Model file for the job. Use its own axes, mm. A direction names the side the tool comes from. Give positions to 0.01 mm unless a question says otherwise; leave off trailing zeros. Write each loop counter-clockwise with the first axis right and the second up, starting at its lowest first coordinate (ties: lowest second). Pieces come first, ordered by that corner, then holes. Notation, with made-up numbers: (0.25, 38.5) - (30.25, 38.5) arc R14 ccw to (30.25, 42.5) - close; hole circle Ø4 at (-5.75, 84). An arc over 180 degrees is marked (long way). One line per item, written item: value. Start each with the question number.
(1) Cut at B-B, the plane x = 34. List the corners of the cut face in (y, z), and give its area (3 significant figures).
(2) 3-axis set-ups, long thin cutter, end or side, ignore diameter. For faces 1 (the face through (86, 73, 3)), 2 (the face through (46.5, -9, 3)), 3 (the face through (69, -25, 3)), 4 (the face through (76, 88, 3)): which of +Z, -Z, +X, -X, +Y, -Y reach the whole face in a straight line?
(3) Cut at C-C, the plane y = 43. List the corners of the cut face in (x, z).
(4) Probe L1, parallel to Y at x = 78, z = 5.3; L2, parallel to X at y = -9, z = 1.35; L3, parallel to X at y = 76.5, z = 3.55. List the from-to ranges inside material, lowest first.
(5) Mould opens along X. For faces 5 (the face through (36.09, 29.32, 2.96)), 6 (the face through (59, 38, 6)), 7 (the face through (81.1, 81, 3)) say: pulls with the +X half, pulls with the -X half, needs draft (parallel to the pull), parting line crosses it, or undercut.
(6) Drop flat-ended pins along their axis: P1, Ø12, axis at x = 82, y = -8.5, coming from the -Z side; P2, Ø10, axis at x = 61, y = 18.5, coming from the -Z side; P3, Ø3, axis at y = 79.5, z = 4.5, coming from the -X side; P4, Ø1.8, axis at y = -5, z = 2, coming from the -X side. Give the stop position or say it passes through.
(7) Cut at A-A, the plane z = 4.45. List the corners of the cut face in (x, y).
from build123d import *

# Parameters (mm, degrees)
BOSS_EXTRU_1_DEPTH = 6
FILLET1_R          = 5
FILLET1_2_R        = 3
FILLET1_3_R        = 1


with BuildPart() as part:
    # Esquisse1 → Boss.-Extru.1 (new body)
    with BuildSketch(Plane.XY):
        with BuildLine():
            Line((46.5, 0), (46.5, -18))
            Line((46.5, -18), (67, -25))
            Line((67, -25), (71, -25))
            Line((71, -25), (71, 88))
            Line((71, 88), (81.1, 88))
            Line((81.1, 88), (81.1, 73))
            Line((81.1, 73), (91.1, 73))
            Line((91.1, 73), (91.1, 100))
            Line((91.1, 100), (69, 100))
            Line((69, 100), (10.371982926, 45.328489608))
            ThreePointArc((10.371982926, 45.328489608), (36.363080219, 28.982346298), (46.5, 0))
        make_face()
    extrude(amount=BOSS_EXTRU_1_DEPTH)

    # Fillet1
    fillet1_edges = [part.edges().sort_by_distance(p)[0] for p in [
        (69, 100, 3),
    ]]
    fillet(fillet1_edges, radius=FILLET1_R)

    # Fillet1 2
    fillet1_2_edges = [part.edges().sort_by_distance(p)[0] for p in [
        (91.1, 100, 3),
    ]]
    fillet(fillet1_2_edges, radius=FILLET1_2_R)

    # Fillet1 3
    fillet1_3_edges = [part.edges().sort_by_distance(p)[0] for p in [
        (91.1, 73, 3),
        (81.1, 73, 3),
    ]]
    fillet(fillet1_3_edges, radius=FILLET1_3_R)


solid = part.part
Answers follow:
1. outline: (31.72, 0) - (67.36, 0) - (67.36, 6) - (31.72, 6) - close
1. area: 214 mm²
2. face 1: +Z, -Z, +X, -Y
2. face 2: +Z, -Z, -X, -Y
2. face 3: +Z, -Z, +X, -X, -Y
2. face 4: +Z, -Z, -Y
3. outline: (17.7, 0) - (71, 0) - (71, 6) - (17.7, 6) - close
4. L1: y = 88 to 100
4. L2: x = 46.5 to 71
4. L3: x = 43.8 to 71, 81.1 to 91.1
5. face 5: pulls with the -X half
5. face 6: needs draft
5. face 7: undercut
6. P1: passes through
6. P2: stops at z = 0
6. P3: stops at x = 45.41
6. P4: stops at x = 46.5
7. outline: (10.37, 45.33) arc R46.5 cw to (46.5, 0) - (46.5, -18) - (67, -25) - (71, -25) - (71, 88) - (81.1, 88) - (81.1, 74) arc R1 ccw to (82.1, 73) - (90.1, 73) arc R1 ccw to (91.1, 74) - (91.1, 97) arc R3 ccw to (88.1, 100) - (70.97, 100) arc R5 ccw to (67.56, 98.66) - close
